```python
from build123d import *

# Parameters (mm, degrees)
F0_W      = 400
F0_H      = 830
F0_W_2    = 320
F0_H_2    = 400
F0_W_3    = 63.6140084174
F0_H_3    = 310
F0_W_4    = 109.7493757494
F1_DEPTH  = 40
F2_W      = 40
F2_H      = 40
F3_DEPTH  = 400
F5_DEPTH  = 40
F7_W      = 400
F7_H      = 40
F8_DEPTH  = 40
F11_DEPTH = 40
F12_R     = 15
F13_DEPTH = 100
F14_R     = 15
F15_DEPTH = 100


with BuildPart() as f1:
    # F0 (on Front) → F1 (new body)
    with BuildSketch(Plane.XZ):
        with Locations((200, -415)):
            Rectangle(F0_W, F0_H)
        with Locations((200, -590)):
            Rectangle(F0_W_2, F0_H_2, mode=Mode.SUBTRACT)
        with Locations((74.8296116246, -195)):
            Rectangle(F0_W_3, F0_H_3, mode=Mode.SUBTRACT)
        with Locations((201.511303708, -195)):
            Rectangle(F0_W_4, F0_H_3, mode=Mode.SUBTRACT)
        with Locations((328.1929957913, -195)):
            Rectangle(F0_W_3, F0_H_3, mode=Mode.SUBTRACT)
    extrude(amount=F1_DEPTH)

    # F2 (on Front) → F3 (join)
    with BuildSketch(Plane.XZ):
        with Locations((380, -850)):
            Rectangle(F2_W, F2_H)
        with Locations((250, -850)):
            Rectangle(F2_W, F2_H)
        with Locations((150, -850)):
            Rectangle(F2_W, F2_H)
        with Locations((20, -850)):
            Rectangle(F2_W, F2_H)
    extrude(amount=F3_DEPTH)

    # F4 (on Right) → F5 (join)
    with BuildSketch(Plane.YZ):
        Polygon((-40, -430), (-40, -364.6261646075), (-400, -830), (-349.4286550909, -830), align=None)
    extrude(amount=F5_DEPTH)

    # F7 (on offset) → F8 (join)
    with BuildSketch(Plane.XZ.offset(400)):
        with Locations((200, -850)):
            Rectangle(F7_W, F7_H)
    extrude(amount=F8_DEPTH)

    # F10 (on offset) → F11 (join)
    with BuildSketch(Plane.YZ.offset(400)):
        Polygon((-400, -830), (-349.4286550909, -830), (-40, -430), (-40, -364.6261646075), align=None)
    extrude(amount=-F11_DEPTH)

    # F12 (on offset) → F13 (join)
    with BuildSketch(Plane.YZ.offset(400)):
        with Locations((-420, -850)):
            Circle(F12_R)
    extrude(amount=F13_DEPTH)

    # F14 (on Right) → F15 (join)
    with BuildSketch(Plane.YZ):
        with Locations((-420, -850)):
            Circle(F14_R)
    extrude(amount=-F15_DEPTH)


solid = f1.part
```
Read the model definition and answer for the solid it produces. Units are mm, in the model's axes. A direction names the side the tool comes from. Give positions to 0.01 mm unless a question says otherwise; leave off trailing zeros. Order: outer loops, then holes, each group sorted by start corner. A loop starts at its lowest first (then second) coordinate and runs counter-clockwise, first axis right, second up. Notation, with made-up numbers: (-28, 1.25) -> (27, 1.25) arc R16 ccw to (27, 6.25) -> close; hole circle Ø6 at (71.25, 78.5). An arc over 180 degrees is marked (long way). Write item = value, one per line.
1. A cutting plane is placed at A-A, the plane z = -108.5. Write down the section's boundary in (x, y).
Numbers:
outline = (0, -40) -> (43.02, -40) -> (43.02, 0) -> (0, 0) -> close; (106.64, -40) -> (146.64, -40) -> (146.64, 0) -> (106.64, 0) -> close; (256.39, -40) -> (296.39, -40) -> (296.39, 0) -> (256.39, 0) -> close; (360, -40) -> (400, -40) -> (400, 0) -> (360, 0) -> close
2. The mould has two halves that part along Z. Classify faces 5 (the face through (197, -20, 0)), 6 (the face through (286, 0, -332)), 7 (the face through (256.386, -20, -197)), 8 (the face through (242, -217, -870)): +Z half, -Z half, draft (parallel to the pull), parting line (faces both ways), or undercut.
Numbers:
face_5 = +Z half
face_6 = draft
face_7 = undercut
face_8 = -Z half
3. Straight lines are drawn through the part: line 1 along X through (y, z) = (-22, -391.5); line 2 along Z through (x, y) = (39.5, -108.5); line 3 along Y through (x, z) = (374, -116). For each, find the intervals that lie inside material, in ascending order.
Numbers:
line_1 = 0 to 40, 360 to 400
line_2 = -870 to -830, -518.55 to -453.18
line_3 = -40 to 0
4. A cutting plane is placed at C-C, the plane y = -231. Write down the section's boundary in (x, z), and give its area (3 significant figures).
Numbers:
outline = (0, -870) -> (40, -870) -> (40, -830) -> (0, -830) -> close; (0, -676.91) -> (40, -676.91) -> (40, -611.53) -> (0, -611.53) -> close; (130, -870) -> (170, -870) -> (170, -830) -> (130, -830) -> close; (230, -870) -> (270, -870) -> (270, -830) -> (230, -830) -> close; (360, -870) -> (400, -870) -> (400, -830) -> (360, -830) -> close; (360, -676.91) -> (400, -676.91) -> (400, -611.53) -> (360, -611.53) -> close
area = 11,600 mm²
5. Given pin 1 (1 mm diameter, centred on x = 31, y = -75.5, fed in from +Z); pin 2 (20 mm diameter, centred on x = 379.5, y = -250, fed in from +Z); pin 3 (12 mm diameter, centred on x = 87.5, y = -22.5, fed in from -Z), each flat-ended and moving along its own axis, determine where each tip first touches the part or whether it passes through.
Numbers:
pin_1 = -409.87
pin_2 = -623.17
pin_3 = -830
6. A cutting plane is placed at B-B, the plane x = 67. Write down the section's boundary in (y, z), and give its area (3 significant figures).
Numbers:
outline = (-440, -870) -> (-400, -870) -> (-400, -830) -> (-440, -830) -> close; (-40, -830) -> (0, -830) -> (0, -790) -> (-40, -790) -> close; (-40, -390) -> (0, -390) -> (0, -350) -> (-40, -350) -> close; (-40, -40) -> (0, -40) -> (0, 0) -> (-40, 0) -> close
area = 6,400 mm²
7. A cutting plane is placed at D-D, the plane x = 157.5. Write down the section's boundary in (y, z), and give its area (3 significant figures).
Numbers:
outline = (-440, -870) -> (0, -870) -> (0, -790) -> (-40, -790) -> (-40, -830) -> (-440, -830) -> close; (-40, -390) -> (0, -390) -> (0, -350) -> (-40, -350) -> close; (-40, -40) -> (0, -40) -> (0, 0) -> (-40, 0) -> close
area = 22,400 mm²
8. For faces 1 (the face through (286, -40, -192)), 2 (the face through (380, -193, -830)), 3 (the face through (43.023, -20, -197)), 4 (the face through (200, -400, -850)), determine the directions among +Z, -Z, +X, -X, +Y, -Y from which every point of the face is accessible in a straight line to the end or side of a thin tool.
Numbers:
face_1 = +Z, -Y
face_2 = +X, -X
face_3 = +Y, -Y
face_4 = +Z, -Z, +Y
